from build123d import *

# Parameters (mm, degrees)
BOX002_W     = 2.4
BOX002_H     = 24
BOX002_DEPTH = 20
BOX003_W     = 2.4
BOX003_H     = 24
BOX003_DEPTH = 20
BOX004_W     = 2.4
BOX004_H     = 24
BOX004_DEPTH = 20
BOX001_W     = 2.4
BOX001_H     = 24
BOX001_DEPTH = 20
BOX_W        = 33
BOX_H        = 30
BOX_DEPTH    = 22


with BuildPart() as box002:
    # Box002 → Box002 (new body)
    with BuildSketch(Plane(origin=(8, -28, 0), x_dir=(1, 0, 0), z_dir=(0, 0, 1))):
        with Locations((1.2, 12)):
            Rectangle(BOX002_W, BOX002_H)
    extrude(amount=BOX002_DEPTH)


with BuildPart() as box003:
    # Box003 → Box003 (new body)
    with BuildSketch(Plane(origin=(16, -28, 0), x_dir=(1, 0, 0), z_dir=(0, 0, 1))):
        with Locations((1.2, 12)):
            Rectangle(BOX003_W, BOX003_H)
    extrude(amount=BOX003_DEPTH)


with BuildPart() as box004:
    # Box004 → Box004 (new body)
    with BuildSketch(Plane(origin=(24, -28, 0), x_dir=(1, 0, 0), z_dir=(0, 0, 1))):
        with Locations((1.2, 12)):
            Rectangle(BOX004_W, BOX004_H)
    extrude(amount=BOX004_DEPTH)


with BuildPart() as fusion:
    # Box001 → Box001 (new body)
    with BuildSketch(Plane(origin=(0, -28, 0), x_dir=(1, 0, 0), z_dir=(0, 0, 1))):
        with Locations((1.2, 12)):
            Rectangle(BOX001_W, BOX001_H)
    extrude(amount=BOX001_DEPTH)

    # Fusion: union Box002, Box003, Box004
    add(box002.part)
    add(box003.part)
    add(box004.part)


with BuildPart() as fusion_1:
    # Fusion placement: moved
    add(fusion.part.moved(Location((-13.2, 31, 4))))


with BuildPart() as cut:
    # Box → Box (new body)
    with BuildSketch(Plane(origin=(-16.5, 0, 0), x_dir=(1, 0, 0), z_dir=(0, 0, 1))):
        with Locations((16.5, 15)):
            Rectangle(BOX_W, BOX_H)
    extrude(amount=BOX_DEPTH)

    # Cut: cut Fusion
    add(fusion_1.part, mode=Mode.SUBTRACT)


solid = cut.part
The listing builds one solid part. Answer for the finished solid, in the listing's coordinates (mm). A direction names the side the tool comes from. Coordinates: 2 decimals unless noted, no trailing zeros. Write each loop counter-clockwise with the first axis right and the second up, starting at its lowest first coordinate (ties: lowest second). Pieces come first, ordered by that corner, then holes. Notation, with made-up numbers: (61.5, 78) -> (101.5, 78) arc R26 cw to (101.5, 95) -> close; hole circle Ø8 at (56.5, 52.25). An arc over 180 degrees is marked (long way). One line per question, with ' | ' between items.
1. Which of the six approach directions +Z, -Z, +X, -X, +Y, -Y give full straight-line access (tool end or side, diameter ignored) to faces 5 (the flat face through (16.5, 15, 11)), 6 (the flat face through (-12, 15, 4))?
Verdict:
face 5: +Z, -Z, +X, +Y, -Y | face 6: +Z
2. For a pull along Y with two mould halves and no side action, classify faces 1 (the flat face through (0, 0, 11)), 2 (the flat face through (10.8, 15, 13)), 3 (the flat face through (0, 15, 22)), 4 (the flat face through (0, 30, 11)) as released by +Y, released by -Y, zero draft, split by the parting line, or undercut.
Verdict:
face 1: released by -Y | face 2: undercut | face 3: zero draft | face 4: released by +Y
3. Section B-B (y = 21) is taken. Determine the outline of the cut face in (x, z).
Verdict:
outline: (-16.5, 0) -> (16.5, 0) -> (16.5, 22) -> (13.2, 22) -> (13.2, 4) -> (10.8, 4) -> (10.8, 22) -> (5.2, 22) -> (5.2, 4) -> (2.8, 4) -> (2.8, 22) -> (-2.8, 22) -> (-2.8, 4) -> (-5.2, 4) -> (-5.2, 22) -> (-10.8, 22) -> (-10.8, 4) -> (-13.2, 4) -> (-13.2, 22) -> (-16.5, 22) -> close
4. Section A-A (z = 6.25) is taken. Determine the outline of the cut face in (x, y).
Verdict:
outline: (-16.5, 0) -> (16.5, 0) -> (16.5, 30) -> (-16.5, 30) -> close; hole (-13.2, 3) -> (-10.8, 3) -> (-10.8, 27) -> (-13.2, 27) -> close; hole (-5.2, 3) -> (-2.8, 3) -> (-2.8, 27) -> (-5.2, 27) -> close; hole (2.8, 3) -> (5.2, 3) -> (5.2, 27) -> (2.8, 27) -> close; hole (10.8, 3) -> (13.2, 3) -> (13.2, 27) -> (10.8, 27) -> close
5. Given pin 1 Ø1.2 at (x, y) = (-3.5, 16) entering from +Z, flat-ended and moving along its own axis, determine where the tip first touches the part or whether it passes through.
Verdict:
pin 1: stops at z = 4
6. Straight lines are drawn through the part: line 1 (X direction, y = 17, z = 12.75); line 2 (Y direction, x = 13, z = 20.75); line 3 (Z direction, x = -3.5, y = 17.25). For each, find the intervals that lie inside material, in ascending order.
Verdict:
line 1: x = -16.5 to -13.2, -10.8 to -5.2, -2.8 to 2.8, 5.2 to 10.8, 13.2 to 16.5 | line 2: y = 0 to 3, 27 to 30 | line 3: z = 0 to 4
